CAD build for the part. Positions are in the model's coordinates, mm. A direction names the side the tool comes from. Round coordinates to 2 decimals unless told otherwise and drop trailing zeros. Order: outer loops, then holes, each group sorted by start corner. A loop starts at its lowest first (then second) coordinate and runs counter-clockwise, first axis right, second up. Notation, with made-up numbers: M 37.25,88.5 L 86.25,88.5 A24 ccw 86.25,100.5 Z; hole C -39.75,56 d2. An arc over 180 degrees is marked long. Answer as a JSON object with one key per item and string values.
Autodesk Inventor part; units mm, degrees
ref_plane "Work Plane2" through (2, 0, 0) normal (1, 0, 0) x (0, 1, 0)
ref_plane "YZ Plane" through (0, 0, 0) normal (1, 0, 0) x (0, 1, 0)
ref_plane "XZ Plane" through (0, 0, 0) normal (0, 1, 0) x (-1, 0, 0)
ref_plane "Work Plane1" through (55, -127.943, -12.5) normal (1, 0, 0) x (0, 0, -1)
ref_plane "Work Plane2" through (2, 0, 0) normal (1, 0, 0) x (0, 1, 0)
ref_plane "Work Plane8" through (55, 3.2, 4) normal (0, 0, 1) x (1, 0, 0)
sketch "SKbody" plane through (55, 3.2, 4) normal (0, 0, 1) x (1, 0, 0)
  line L0 (0, 10.8) -> (-34, 10.8)
  line L1 (-34, -5.2) -> (0, -5.2)
  line L2 (-34, 10.8) -> (-34, -5.2)
  line L3 (0, -5.2) -> (0, 10.8)
  line L4 (0, -2.2986) -> (0, 7.8986)
  point P0 (-13, 2.8)
  point P1 (0, 2.8)
  dimension "d19" = 34
  dimension "d20" = 13
extrude "EXbody" add sketch "SKbody" along normal blind 22.8
ref_plane "Work Plane6" through (21, -2, 4) normal (-1, 0, 0) x (0, 0, 1)
sketch "SKhole1" plane through (21, -2, 4) normal (-1, 0, 0) x (0, 0, 1)
  line L0 (22.8, 16) -> (22.8, 0)
  circle A0 centre (22.8, 8) radius 6
  point P0 (22.8, 2)
  point P1 (22.8, 14)
  dimension "d11" = 12
extrude "EXhole1" cut sketch "SKhole1" against normal through all contours L0 A0 picked at (20.93, 8.7092)
ref_plane "Work Plane5" through (55, 3.2, 26.8) normal (0, 0, 1) x (1, 0, 0)
sketch "SKplaneref" plane through (55, 3.2, 26.8) normal (0, 0, 1) x (1, 0, 0)
  line L0 (0, 8.8) -> (0, -3.2)
  line L1 (0, 2.8) -> (-2, 2.8)
  dimension "d15" = 2
ref_plane "Work Plane3" through (53, 6, 26.8) normal (-1, 0, 0) x (0, -1, 0)
sketch "SKhole2" plane through (53, 6, 26.8) normal (-1, 0, 0) x (0, -1, 0)
  arc A0 (-6, 0) -> (6, 0) centre (0, 0) ccw
  circle A1 centre (0, 0) radius 7
  point P0 (6, -26.8)
  dimension "d16" = 14
extrude "EXhole2" cut sketch "SKhole2" along normal blind 22
ref_plane "Work Plane7" through (21, 14, 4) normal (0, 1, 0) x (1, 0, 0)
sketch "SKziptiehole" plane through (21, 14, 4) normal (0, 1, 0) x (1, 0, 0)
  line L0 (34, -22.8) -> (0, -22.8)
  line L1 (0, 0) -> (0, -22.8)
  point P0 (8, -10.8)
  dimension "d42" = 12
  dimension "d43" = 8
hole "Hziptiehole" at (29, 14, 14.8) direction (0, -1, 0) diameter 4 end through all
fillet "Fillet1" radius 0.5 12 edges at (21, 14, 15.4) (38, 14, 26.8) (38, -2, 26.8) (21, -2, 15.4) (55, 14, 15.4) (55, -2, 15.4) (55, 6, 20.8) (21, 6, 20.8) (26, 0, 26.8) (26, 12, 26.8) (53, 6, 20.8) (31, 6, 20.8)
properties part number "thermoMETER_mount"
Item 1: 3-axis set-ups, long thin cutter, end or side, ignore diameter. For faces 1 (the flat face through (55, 6, 13)), 2 (the cylindrical face through (42.15, 5.85, 19.8)): which of +Z, -Z, +X, -X, +Y, -Y reach the whole face in a straight line?
Worked answers:
{"face 1": "+Z, -Z, +X, +Y, -Y", "face 2": "+Z"}
Item 2: Wall check: line 1 along X through (y, z) = (2, 14.8); line 2 along Z through (x, y) = (29, 5.75); line 3 along Z through (x, y) = (29, 10.5). Give the ranges that are in metal, low to high. Write a range as [from, to].
Worked answers:
{"line 1": "x = [21, 27], [31, 55]", "line 2": "z = [4, 12.8], [16.8, 20.81]", "line 3": "z = [4, 12.8], [16.8, 22.83]"}
Item 3: Drop flat-ended pins along their axis: pin 1 Ø1 at (x, y) = (33, 4.5) entering from +Z; pin 2 Ø2 at (x, y) = (25.5, 5) entering from +Z; pin 3 Ø3 at (x, y) = (42.5, 9) entering from +Z. Give the stop position or say it passes through.
Worked answers:
{"pin 1": "stops at z = 20.09", "pin 2": "stops at z = 21.14", "pin 3": "stops at z = 21.44"}
Item 4: Saw through at A-A on z = 14.8. List the corners of the cut face in (x, y).
Worked answers:
{"outline": "M 21,-1.5 A0.5 ccw 21.5,-2 L 27,-2 L 27,14 L 21.5,14 A0.5 ccw 21,13.5 Z; M 31,-2 L 54.5,-2 A0.5 ccw 55,-1.5 L 55,13.5 A0.5 ccw 54.5,14 L 31,14 Z"}
Item 5: Two-plate mould, pull along Y, no slides. Class faces 3 (the flat face through (38, 6, 4)), 4 (the flat face through (38, 14, 15)), 5 (the flat face through (31, 6, 20)): released by +Y, released by -Y, zero draft, split by the parting line, or undercut.
Worked answers:
{"face 3": "zero draft", "face 4": "released by +Y", "face 5": "undercut"}
Item 6: Saw through at C-C on y = 6. List the corners of the cut face in (x, z).
Worked answers:
{"outline": "M 21,4 L 55,4 L 55,20.3 A0.5 ccw 54.5,20.8 L 53.5,20.8 A0.5 ccw 53,20.3 L 53,19.8 L 31,19.8 L 31,20.3 A0.5 ccw 30.5,20.8 L 21.5,20.8 A0.5 ccw 21,20.3 Z; hole C 29,14.8 d4"}
Item 7: Saw through at B-B on x = 29. List the corners of the cut face in (y, z).
Worked answers:
{"outline": "M -2,4 L 14,4 L 14,12.8 L -2,12.8 Z; M -2,16.8 L 14,16.8 L 14,26.3 A0.5 ccw 13.5,26.8 L 12.48,26.8 A0.5 ccw 11.98,26.34 A6 cw 0.02,26.34 A0.5 ccw -0.48,26.8 L -1.5,26.8 A0.5 ccw -2,26.3 Z"}
Item 8: Saw through at D-D on x = 34.5. List the corners of the cut face in (y, z).
Worked answers:
{"outline": "M -2,4 L 14,4 L 14,26.3 A0.5 ccw 13.5,26.8 L 13,26.8 A7 cw -1,26.8 L -1.5,26.8 A0.5 ccw -2,26.3 Z"}
